Geometry: final body of the model. Coordinates: model frame, mm. A direction names the side the tool comes from. Coordinates: 2 decimals unless noted, no trailing zeros. Order: outer loops, then holes, each group sorted by start corner. A loop starts at its lowest first (then second) coordinate and runs counter-clockwise, first axis right, second up. Notation, with made-up numbers: (-20, 14) -> (10, 14) arc R12 cw to (10, 21) -> close; hole circle Ø3 at (26.5, 1.25). An arc over 180 degrees is marked (long way). Answer in a Markdown table with one row per item. Add a question column.
1) Pull-direction query (Y, two-part tool) for faces 5 (the face through (37, 47, 15)), 6 (the face through (37, 6, 15)), 7 (the face through (161, 26, 5.5)), 8 (the face through (115, 26, -0.75)); classes: +Y half, -Y half, draft (parallel to the pull), parting line (faces both ways), or undercut.
2) Ray query, line 1 (Y direction, x = -97.5, z = 3.75); line 2 (Z direction, x = 109.5, y = 11.5); line 3 (Z direction, x = 6, y = 42). Return the intervals inside material, ascending. Write a range as from..to.
3) Contact query for flat-ended pins moving along their axis: P1, Ø1.5, axis at y = 34.5, z = 7.5, coming from the -X side; P2, Ø7.5, axis at y = 20.5, z = 3.5, coming from the -X side; P3, Ø6, axis at x = 125, y = 25.5, coming from the +Z side; P4, Ø0.8, axis at x = 147, y = 18, coming from the +Z side. Output: stop coordinate, or through.
4) Section query B-B on x = 82.5. Return the cut outline in (y, z).
5) Section query A-A on x = 34. Return the cut outline in (y, z), then the cut area to 3 significant figures.
6) Set-up query: faces 1 (the face through (-4, 26, 10)), 2 (the face through (-4.87, 26.79, 4.68)), 3 (the face through (115, 26, 1.75)), 4 (the face through (54.57, 26.77, 12)). Return all of +Z, -Z, +X, -X, +Y, -Y with unobstructed straight access to the full face (end or side cutting, diameter ignored); none if empty.
7) Section query C-C on x = -91. Return the cut outline in (y, z).
```python
from build123d import *

# Parameters (mm, degrees)
SKETCH037_W                               = 2
SKETCH037_H                               = 41
EXTRUDE036_DEPTH                          = 1
SKETCH032_AS_DRAWN_W                      = 36.96
SKETCH032_AS_DRAWN_H                      = 13
EXTRUDE030_DEPTH                          = 2
EXTRUDE030_ONTO_SKETCH032_ROLL_ANGLE      = 0.005477
EXTRUDE030_ONTO_SKETCH032_PITCH_ANGLE     = -0.011215
EXTRUDE030_ONTO_SKETCH032_PLACEMENT_ANGLE = 89.994139
SKETCH031_W                               = 37
SKETCH031_H                               = 2.5
EXTRUDE029_DEPTH                          = 120
SKETCH030_W                               = 56
SKETCH030_H                               = 13.5
EXTRUDE028_DEPTH                          = 41
FILLET009_R                               = 5
FILLET010_R                               = 1.75
SKETCH036_W                               = 120
SKETCH036_H                               = 8
EXTRUDE035_DEPTH                          = 2
FILLET011_R                               = 1
FILLET012_R                               = 1
FILLET013_R                               = 0.25
FILLET014_R                               = 1


with BuildPart() as velcroborder:
    # Sketch037 → Extrude036 (new body)
    with BuildSketch(Plane.XY.offset(5.5)):
        with Locations((174, 26.5)):
            Rectangle(SKETCH037_W, SKETCH037_H)
        with Locations((147, 26.5)):
            Rectangle(SKETCH037_W, SKETCH037_H)
    extrude(amount=EXTRUDE036_DEPTH)


with BuildPart() as sensorcuts:
    # Sketch032 as drawn → Extrude030 (new)
    with BuildSketch(Plane.XY):
        with Locations((-0.07, -91)):
            Rectangle(SKETCH032_AS_DRAWN_W, SKETCH032_AS_DRAWN_H)
    extrude(amount=EXTRUDE030_DEPTH)


with BuildPart() as sensorcuts_1:
    # Extrude030 onto Sketch032 roll: moved
    add(sensorcuts.part.rotate(Axis((0, 0, 0), (1, 0, 0)), EXTRUDE030_ONTO_SKETCH032_ROLL_ANGLE))


with BuildPart() as sensorcuts_2:
    # Extrude030 onto Sketch032 pitch: moved
    add(sensorcuts_1.part.rotate(Axis((0, 0, 0), (0, 1, 0)), EXTRUDE030_ONTO_SKETCH032_PITCH_ANGLE))


with BuildPart() as sensorcuts_3:
    # Extrude030 onto Sketch032 placement: moved
    add(sensorcuts_2.part.moved(Location((50.768112, 26.489725, 2.608705))).rotate(Axis((50.768112, 26.489725, 2.608705), (0, 0, 1)), EXTRUDE030_ONTO_SKETCH032_PLACEMENT_ANGLE))


with BuildPart() as sensorcuts_4:
    # Extrude030 placement: moved
    add(sensorcuts_3.part.moved(Location((0, 0, -4))))


with BuildPart() as extrude029:
    # Sketch031 → Extrude029 (new body)
    with BuildSketch(Plane.YZ.offset(56)):
        with Locations((26.412533, 0.5)):
            Rectangle(SKETCH031_W, SKETCH031_H)
    extrude(amount=EXTRUDE029_DEPTH)


with BuildPart() as band003:
    # Sketch030 → Extrude028 (new body)
    with BuildSketch(Plane.XZ.offset(-6)):
        Polygon((175, 5.5), (60, 5.5), (60, 17.5), (-4, 17.5), (-4, 2.5), (-122, 2.5), (-122, -2.5), (175, -2.5), align=None)
        with Locations((28, 6.75)):
            Rectangle(SKETCH030_W, SKETCH030_H, mode=Mode.SUBTRACT)
    extrude(amount=-EXTRUDE028_DEPTH)

    # Cut002: cut Extrude029
    add(extrude029.part, mode=Mode.SUBTRACT)

    # Cut003: cut sensorCuts
    add(sensorcuts_4.part, mode=Mode.SUBTRACT)

    # Fillet009
    fillet009_edges = [band003.edges().sort_by_distance(p)[0] for p in [
        (60, 26.5, 5.5),
        (60, 26.5, 17.5),
        (-4, 26.5, 17.5),
        (-4, 26.5, 2.5),
        (0, 26.5, 0),
        (0, 26.5, 13.5),
        (56, 26.5, 13.5),
    ]]
    fillet(fillet009_edges, radius=FILLET009_R)

    # Fillet010
    fillet010_edges = [band003.edges().sort_by_distance(p)[0] for p in [
        (56, 6.956266, 0),
        (56, 45.956266, 0),
    ]]
    fillet(fillet010_edges, radius=FILLET010_R)


with BuildPart() as fillet014:
    # Sketch036 → Extrude035 (new body)
    with BuildSketch(Plane.XY.offset(2.5)):
        with Locations((-62, 43)):
            Rectangle(SKETCH036_W, SKETCH036_H)
        with Locations((-62, 10)):
            Rectangle(SKETCH036_W, SKETCH036_H)
    extrude(amount=EXTRUDE035_DEPTH)

    # Fusion011: union velcroBorder, band003
    add(velcroborder.part)
    add(band003.part)

    # Fillet011
    fillet011_edges = [fillet014.edges().sort_by_distance(p)[0] for p in [
        (56, 26.412533, 1.75),
    ]]
    fillet(fillet011_edges, radius=FILLET011_R)

    # Fillet012
    fillet012_edges = [fillet014.edges().sort_by_distance(p)[0] for p in [
        (26.5, 6, -2.5),
        (26.5, 47, -2.5),
        (-63.5, 6, 4.5),
        (-63.5, 47, 4.5),
        (-63.5, 39, 4.5),
        (-63.5, 14, 4.5),
    ]]
    fillet(fillet012_edges, radius=FILLET012_R)

    # Fillet013
    fillet013_edges = [fillet014.edges().sort_by_distance(p)[0] for p in [
        (175, 26.5, 6.5),
        (173, 26.5, 6.5),
        (148, 26.5, 6.5),
        (146, 26.5, 6.5),
    ]]
    fillet(fillet013_edges, radius=FILLET013_R)

    # Fillet014
    fillet014_edges = [fillet014.edges().sort_by_distance(p)[0] for p in [
        (28, 6, 13.5),
        (28, 47, 13.5),
    ]]
    fillet(fillet014_edges, radius=FILLET014_R)


solid = fillet014.part
```
Result:
| question | item | result |
|---|---|---|
| 1 | face 5 | +Y half |
| 1 | face 6 | -Y half |
| 1 | face 7 | draft |
| 1 | face 8 | undercut |
| 2 | line 1 | 6.03..13.97, 39.03..46.97 |
| 2 | line 2 | -2.5..-0.75, 1.75..5.5 |
| 2 | line 3 | -2.5..0, 13.5..17.5 |
| 3 | P1 | x = -4.06 |
| 3 | P2 | x = -122 |
| 3 | P3 | z = 5.5 |
| 3 | P4 | z = 6.5 |
| 4 | outline | (6, -1.5) arc R1 ccw to (7, -2.5) -> (46, -2.5) arc R1 ccw to (47, -1.5) -> (47, 5.5) -> (6, 5.5) -> close; hole (7.91, -0.75) -> (44.91, -0.75) -> (44.91, 1.75) -> (7.91, 1.75) -> close |
| 5 | outline | (6, -1.5) arc R1 ccw to (7, -2.5) -> (46, -2.5) arc R1 ccw to (47, -1.5) -> (47, -1) arc R1 ccw to (46, 0) -> (7, 0) arc R1 ccw to (6, -1) -> close; (6, 14.5) arc R1 ccw to (7, 13.5) -> (46, 13.5) arc R1 ccw to (47, 14.5) -> (47, 17.5) -> (6, 17.5) -> close |
| 5 | area | 265 mm2 |
| 6 | face 1 | +Z, -X, +Y, -Y |
| 6 | face 2 | +Z, -X |
| 6 | face 3 | +X |
| 6 | face 4 | +Y, -Y |
| 7 | outline | (6, -1.5) arc R1 ccw to (7, -2.5) -> (46, -2.5) arc R1 ccw to (47, -1.5) -> (47, 3.5) arc R1 ccw to (46, 4.5) -> (40, 4.5) arc R1 ccw to (39, 3.5) -> (39, 2.5) -> (14, 2.5) -> (14, 3.5) arc R1 ccw to (13, 4.5) -> (7, 4.5) arc R1 ccw to (6, 3.5) -> close |
